from build123d import *

# Parameters (mm, degrees)
SKETCH_1_R      = 2.5
EXTRUDE_1_DEPTH = 17
EXTRUDE_2_DEPTH = 3.5
FILLET_1_R      = 1


with BuildPart() as part:
    # Эскиз1 → Вытянуть1 (new body)
    with BuildSketch(Plane(origin=(0, 0, 0), x_dir=(1, 0, 0), z_dir=(0, 1, 0))):
        with Locations(Location((0, 0, 0), (0, 0, 270))):
            Circle(SKETCH_1_R)
    extrude(amount=EXTRUDE_1_DEPTH)

    # Эскиз2 → Вытянуть2 (add)
    with BuildSketch(Plane(origin=(0, 17, 0), x_dir=(1, 0, 0), z_dir=(0, 1, 0))):
        Polygon((3.621435705, -2.866799046), (4.293438654, 1.702855795), (0.672002949, 4.569654841), (-3.621435705, 2.866799046), (-4.293438654, -1.702855795), (-0.672002949, -4.569654841), align=None)
    extrude(amount=EXTRUDE_2_DEPTH)

    # Скругление1
    fillet_1_edges = [part.edges().sort_by_distance(p)[0] for p in [
        (1.474716378, 20.5, 3.718226944),
        (3.957437179, 20.5, 0.581971625),
        (2.482720801, 20.5, -3.136255318),
        (-1.474716378, 20.5, -3.718226944),
        (-3.957437179, 20.5, -0.581971625),
        (-2.482720801, 20.5, 3.136255318),
    ]]
    fillet(fillet_1_edges, radius=FILLET_1_R)


solid = part.part
The listing builds one solid part. Answer for the finished solid, in the listing's coordinates (mm). A direction names the side the tool comes from. Round coordinates to 2 decimals unless told otherwise and drop trailing zeros. Write each loop counter-clockwise with the first axis right and the second up, starting at its lowest first coordinate (ties: lowest second). Pieces come first, ordered by that corner, then holes. Notation, with made-up numbers: (79.5, -39) - (105.5, -39) arc R13 ccw to (105.5, -14) - close; hole circle Ø1 at (-35.75, 58). An arc over 180 degrees is marked (long way). Use a Markdown table: item, result. Add a question column.
1. The part is cut by section A-A (y = 19). Write down the section's boundary in (x, z), and give its area (3 significant figures).
2. The part is cut by section B-B (y = 15.75). Write down the section's boundary in (x, z).
3. A tool of negligible diameter and unlimited length cuts with its end or side. For faces 1 (the face through (-2, 17, -2)), 2 (the face through (1.4, 20.2, 3.44)), from which of +Z, -Z, +X, -X, +Y, -Y can it reach the whole face along a straight path? Write none if from no direction.
4. Consider line 1 (Y direction, x = 3, z = 0.75); line 2 (X direction, y = 2.5, z = 0.5); line 3 (X direction, y = 5.5, z = -2.25). Determine where each line is inside the solid, lowest interval first.
5. Flat-ended cylindrical pins translate along their axes: P1, Ø2, axis at x = 2.5, y = 5, coming from the +Z side; P2, Ø2, axis at x = 1.5, y = 15, coming from the +Z side; P3, Ø4, axis at y = 2.5, z = -1, coming from the -X side. Find the tip coordinate at first contact, or state that the pin passes through.
Reported:
| question | item | result |
|---|---|---|
| 1 | outline | (-4.29, 1.7) - (-3.62, -2.87) - (0.67, -4.57) - (4.29, -1.7) - (3.62, 2.87) - (-0.67, 4.57) - close |
| 1 | area | 55.4 mm^2 |
| 2 | outline | circle Ø5 at (0, 0) |
| 3 | face 1 | -Y |
| 3 | face 2 | +Z, +X, +Y |
| 4 | line 1 | 17 to 20.5 |
| 4 | line 2 | -2.45 to 2.45 |
| 4 | line 3 | -1.09 to 1.09 |
| 5 | P1 | z = 2 |
| 5 | P2 | z = 2.45 |
| 5 | P3 | x = -2.5 |
